```python
from build123d import *

# Parameters (mm, degrees)
SKIZZE2_W                            = 130
SKIZZE2_H                            = 30
SKIZZE2_R                            = 2.4
AUFSATZ_LINEAR_AUSTRAGEN1_DEPTH      = 11
AUFSATZ_LINEAR_AUSTRAGEN1_DEPTH_BACK = 11
SCHNITT_LINEAR_AUSTRAGEN1_REACH      = 32


with BuildPart() as part:
    # Skizze2 → Aufsatz-Linear austragen1 (new body, two sides)
    with BuildSketch(Plane(origin=(0, 0, 0), x_dir=(1, 0, 0), z_dir=(0, 1, 0))) as aufsatz_linear_austragen1_sk:
        Rectangle(SKIZZE2_W, SKIZZE2_H)
        with Locations((-53, -7.5)):
            Circle(SKIZZE2_R, mode=Mode.SUBTRACT)
        with Locations((-53, 7.5)):
            Circle(SKIZZE2_R, mode=Mode.SUBTRACT)
        with Locations((53, -7.5)):
            Circle(SKIZZE2_R, mode=Mode.SUBTRACT)
        with Locations((53, 7.5)):
            Circle(SKIZZE2_R, mode=Mode.SUBTRACT)
    extrude(amount=AUFSATZ_LINEAR_AUSTRAGEN1_DEPTH)
    extrude(aufsatz_linear_austragen1_sk.sketch, amount=-AUFSATZ_LINEAR_AUSTRAGEN1_DEPTH_BACK)

    # Skizze5 → Schnitt-Linear austragen1 (cut, up to next)
    with BuildSketch(Plane.XY.offset(15), mode=Mode.PRIVATE) as schnitt_linear_austragen1_sk1:
        with BuildLine():
            Line((-25.101020514, 5), (25.101020514, 5))
            ThreePointArc((25.101020514, 5), (37, 0), (25.101020514, -5))
            Line((25.101020514, -5), (-25.101020514, -5))
            ThreePointArc((-25.101020514, -5), (-37, 0), (-25.101020514, 5))
        make_face()
    schnitt_linear_austragen1_tool1 = extrude(schnitt_linear_austragen1_sk1.sketch, amount=-SCHNITT_LINEAR_AUSTRAGEN1_REACH, mode=Mode.PRIVATE) & part.part
    add(schnitt_linear_austragen1_tool1.solids().sort_by_distance((0, 0, 15))[0], mode=Mode.SUBTRACT)


solid = part.part
```
Part model, mm, in its own coordinate system. A direction names the side the tool comes from. Give positions to 0.01 mm unless a question says otherwise; leave off trailing zeros. Order: outer loops, then holes, each group sorted by start corner. A loop starts at its lowest first (then second) coordinate and runs counter-clockwise, first axis right, second up. Notation, with made-up numbers: M 65.25,-30.5 L 109.25,-30.5 A12 ccw 109.25,-7.5 Z; hole C -31,11.25 d8. An arc over 180 degrees is marked long. Use a Markdown table: item, result. Add a question column.
(1) Saw through at B-B, the plane x = 3. Give the cut face in (y, z).
(2) 3-axis set-ups, long thin cutter, end or side, ignore diameter. For faces 1 (the face through (-1, 7, -15)), 2 (the face through (0, -5, 0)): which of +Z, -Z, +X, -X, +Y, -Y reach the whole face in a straight line?
(3) Saw through at C-C, the plane y = 2.75. Give the cut face in (x, z).
(4) Saw through at D-D, the plane x = 30. Give the cut face in (y, z).
(5) Mould opens along X. For faces 3 (the face through (0, 5, 0)), 4 (the face through (-1, 11, 0)), 5 (the face through (65, 0, 0)) say: +X half, -X half, draft (parallel to the pull), parting line (faces both ways), or undercut.
(6) Saw through at A-A, the plane z = -7.5. Give the cut face in (x, y), and give its area (3 significant figures).
(7) Probe line 1 along Z through (x, y) = (53, -5); line 2 along X through (y, z) = (-8.5, -7.5); line 3 along X through (y, z) = (0, 8.5). List the from-to ranges inside material, lowest first. Write a range as [from, to].
Answer key:
| question | item | result |
|---|---|---|
| 1 | outline | M -11,-15 L -5,-15 L -5,15 L -11,15 Z; M 5,-15 L 11,-15 L 11,15 L 5,15 Z |
| 2 | face 1 | -Z, +X, -X, +Y, -Y |
| 2 | face 2 | +Z, -Z |
| 3 | outline | M -65,-15 L -36.44,-15 L -36.44,15 L -65,15 Z; M 36.44,-15 L 65,-15 L 65,15 L 36.44,15 Z; hole C -53,-7.5 d4.8; hole C -53,7.5 d4.8; hole C 53,-7.5 d4.8; hole C 53,7.5 d4.8 |
| 4 | outline | M -11,-15 L -7,-15 L -7,15 L -11,15 Z; M 7,-15 L 11,-15 L 11,15 L 7,15 Z |
| 5 | face 3 | undercut |
| 5 | face 4 | draft |
| 5 | face 5 | +X half |
| 6 | outline | M -65,-11 L -55.4,-11 L -55.4,11 L -65,11 Z; M -50.6,-11 L 50.6,-11 L 50.6,11 L -50.6,11 Z; M 55.4,-11 L 65,-11 L 65,11 L 55.4,11 Z; hole M -25.1,-5 L 25.1,-5 A7 ccw long 25.1,5 L -25.1,5 A7 ccw long Z |
| 6 | area | 1,870 mm^2 |
| 7 | line 1 | [-15, -9.9], [-5.1, 5.1], [9.9, 15] |
| 7 | line 2 | [-65, -55.4], [-50.6, 50.6], [55.4, 65] |
| 7 | line 3 | [-65, -55.18], [-50.82, -37], [37, 50.82], [55.18, 65] |
